Answer from the drawing. Dimensions are ordinates in mm from the lowest x, y and z of the part. Coordinates: 2 decimals unless noted, no trailing zeros. Order: outer loops, then holes, each group sorted by start corner. A loop starts at its lowest first (then second) coordinate and runs counter-clockwise, first axis right, second up. Notation, with made-up numbers: (60.25, -37) - (115.25, -37) arc R20 ccw to (115.25, -20) - close; hole circle Ø7 at (36, 0). An arc over 180 degrees is marked (long way). Use a Markdown table: item, result. Add a question column.
Item 1: The part is cut by section A-A, the plane z = 20. Give the vertices of the cut face in (x, y), then the cut area to 3 significant figures.
Item 2: The part is cut by section D-D, the plane z = 93.5. Give the vertices of the cut face in (x, y), then the cut area to 3 significant figures.
Item 3: The part is cut by section B-B, the plane y = 1.75. Give the vertices of the cut face in (x, z).
Item 4: Flat-ended cylindrical pins translate along their axes: P1, Ø11.5, axis at x = 15, z = 80, coming from the -Y side; P2, Ø8, axis at x = 15, z = 20, coming from the -Y side. Find the tip coordinate at first contact, or state that the pin passes through.
Item 5: The part is cut by section C-C, the plane z = 77.5. Give the vertices of the cut face in (x, y).
Item 6: Find the intervals of material crossed by line 1 along X through (y, z) = (7.5, 20); line 2 along X through (y, z) = (3.75, 78.5); line 3 along Z through (x, y) = (140, 4.5), in increasing order.
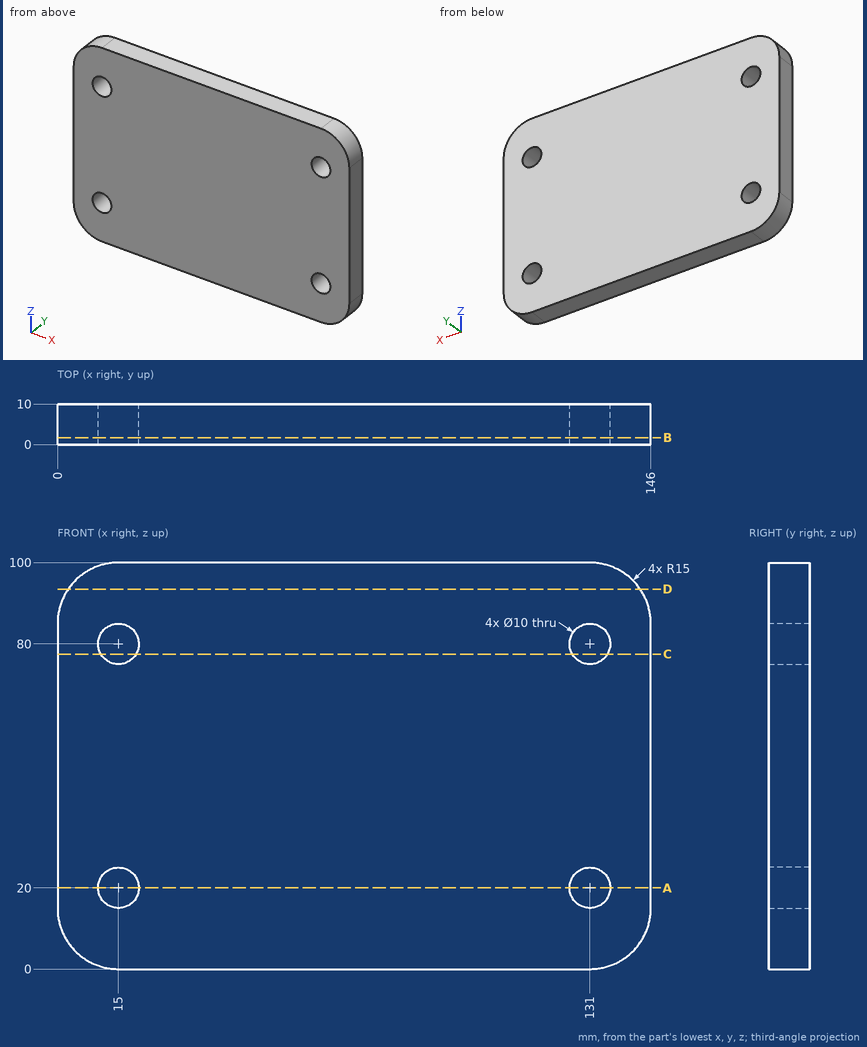
Solution:
| question | item | result |
|---|---|---|
| 1 | outline | (0, 0) - (10, 0) - (10, 10) - (0, 10) - close; (20, 0) - (126, 0) - (126, 10) - (20, 10) - close; (136, 0) - (146, 0) - (146, 10) - (136, 10) - close |
| 1 | area | 1,260 mm2 |
| 2 | outline | (2.64, 0) - (143.36, 0) - (143.36, 10) - (2.64, 10) - close |
| 2 | area | 1,410 mm2 |
| 3 | outline | (0, 15) arc R15 ccw to (15, 0) - (131, 0) arc R15 ccw to (146, 15) - (146, 85) arc R15 ccw to (131, 100) - (15, 100) arc R15 ccw to (0, 85) - close; hole circle Ø10 at (15, 20); hole circle Ø10 at (15, 80); hole circle Ø10 at (131, 20); hole circle Ø10 at (131, 80) |
| 4 | P1 | stops at y = 0 |
| 4 | P2 | passes through |
| 5 | outline | (0, 0) - (10.67, 0) - (10.67, 10) - (0, 10) - close; (19.33, 0) - (126.67, 0) - (126.67, 10) - (19.33, 10) - close; (135.33, 0) - (146, 0) - (146, 10) - (135.33, 10) - close |
| 6 | line 1 | x = 0 to 10, 20 to 126, 136 to 146 |
| 6 | line 2 | x = 0 to 10.23, 19.77 to 126.23, 135.77 to 146 |
| 6 | line 3 | z = 3 to 97 |
